For this review, take the finished solid that the model builds, in its own axes (mm). Give positions to 0.01 mm unless a question says otherwise; leave off trailing zeros. Write each loop counter-clockwise with the first axis right and the second up, starting at its lowest first coordinate (ties: lowest second). Pieces come first, ordered by that corner, then holes. Notation, with made-up numbers: (3.25, 15) -> (45.25, 15) arc R20 cw to (45.25, 24) -> close; hole circle Ø4 at (-38, 61.25). An arc over 180 degrees is marked (long way). Write item = value, one per line.
```python
from build123d import *

# Parameters (mm, degrees)
F0_W     = 12.7
F0_H     = 44.45
F1_DEPTH = 9.525
F2_R     = 1.6002
F3_DEPTH = 25.4
F5_DEPTH = 25.4


with BuildPart() as f1:
    # F0 (on Front) → F1 (new body)
    with BuildSketch(Plane.XZ):
        Rectangle(F0_W, F0_H)
    extrude(amount=F1_DEPTH)

    # F2 (on face) → F3 (cut)
    with BuildSketch(Plane.XY.offset(22.225)):
        with Locations((0, -4.7625)):
            Circle(F2_R)
    extrude(amount=-F3_DEPTH, mode=Mode.SUBTRACT)

    # F4 (on face) → F5 (cut)
    with BuildSketch(Plane.XZ.offset(9.525)):
        Polygon((4.7625, -22.225), (4.493098, 9.523857), (-5.031902, 9.523857), (-4.7625, -22.225), align=None)
    extrude(amount=-F5_DEPTH, mode=Mode.SUBTRACT)


solid = f1.part
```
(1) Take a section at C-C (z = -13.5). Write out the cut boundary in (x, y) (3 decimals), plus the area to 3 significant figures.
Answers below:
outline = (-6.35, -9.525) -> (-4.837, -9.525) -> (-4.837, 0) -> (-6.35, 0) -> close; (4.688, -9.525) -> (6.35, -9.525) -> (6.35, 0) -> (4.688, 0) -> close
area = 30.2 mm^2
(2) Take a section at D-D (x = -2). Write out the cut boundary in (y, z) (3 decimals), plus the area to 3 significant figures.
Answers below:
outline = (-9.525, 9.524) -> (0, 9.524) -> (0, 22.225) -> (-9.525, 22.225) -> close
area = 121 mm^2
(3) Take a section at A-A (x = 0). Write out the cut boundary in (y, z) (3 decimals).
Answers below:
outline = (-9.525, 9.524) -> (-6.363, 9.524) -> (-6.363, 22.225) -> (-9.525, 22.225) -> close; (-3.162, 9.524) -> (0, 9.524) -> (0, 22.225) -> (-3.162, 22.225) -> close
(4) For pin 1 (3 mm diameter, centred on x = -2.5, y = -2.5, fed in from -Z), flat-tipped, find the tip position at first contact; note if it passes through.
Answers below:
pin_1 = 9.52
(5) To check wall thickness, follow probe 1 along Y at (x, z) = (0, 16) (3 decimals); probe 2 along Z at (x, y) = (-0.25, -1.25) (3 decimals); probe 3 along X at (y, z) = (-0.25, -1). State the ranges of each line that lie inside material, in increasing order.
Answers below:
probe_1 = -9.525 to -6.363, -3.162 to 0
probe_2 = 9.524 to 22.225
probe_3 = -6.35 to -4.94, 4.58 to 6.35
(6) The part is to be moulded in two halves that separate along X. For faces 1 (the face through (-2, -5, 9.524)), 2 (the face through (-6.35, -5, 0)), 3 (the face through (0, -9.525, 10)), say which applies: released by +X, released by -X, zero draft, split by the parting line, or undercut.
Answers below:
face_1 = undercut
face_2 = released by -X
face_3 = zero draft
